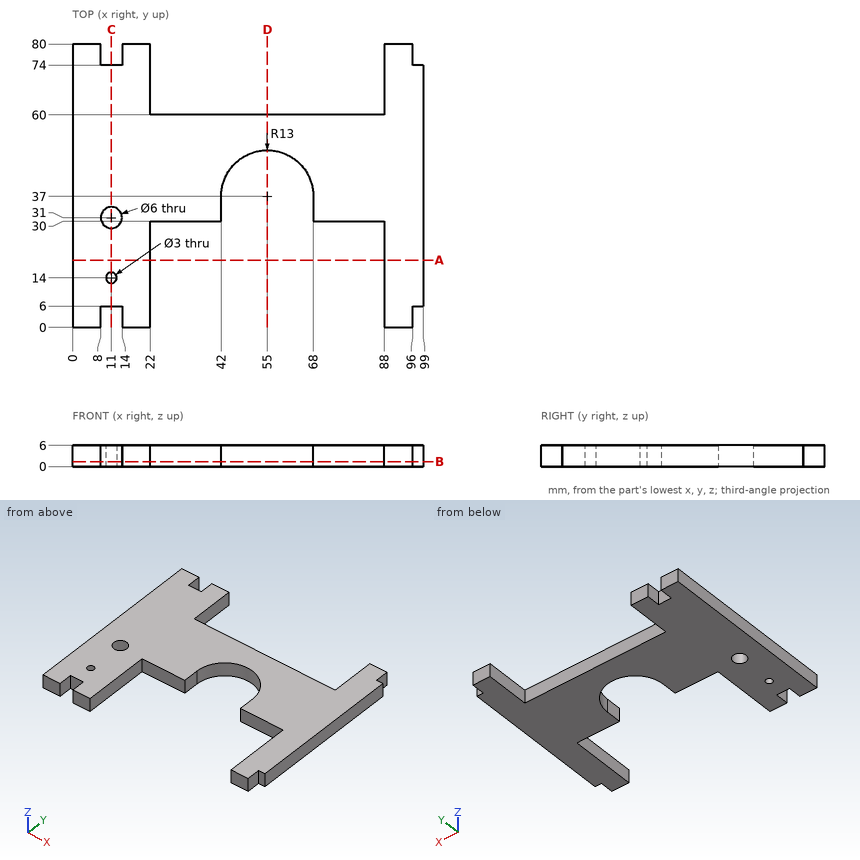
Verification items for this drawing (mm, ordinates from the low corner). Coordinates: 2 decimals unless noted, no trailing zeros. Loops run counter-clockwise (first coordinate to the right, second up) from the corner with the lowest first, then second, coordinate; pieces in that order, holes last. Notation, with made-up numbers: (44.25, -21.75) - (88.25, -21.75) arc R19 ccw to (88.25, -1.75) - close; hole circle Ø9 at (59.25, 23.25). An arc over 180 degrees is marked (long way). Answer as a JSON object with one key per item and string values.
(1) Cross-section at C-C, the plane x = 11. Record the boundary of the cut face in (y, z), then the cut area to 3 significant figures.
Response:
{"outline": "(6, 0) - (12.5, 0) - (12.5, 6) - (6, 6) - close; (15.5, 0) - (28, 0) - (28, 6) - (15.5, 6) - close; (34, 0) - (74, 0) - (74, 6) - (34, 6) - close", "area": "354 mm²"}
(2) Cross-section at B-B, the plane z = 1.4. Count the separate pieces of the cut face and the enclosed holes in it, then the cut area to 3 significant figures.
Response:
{"separate pieces": "1", "enclosed holes": "2", "area": "4,030 mm²"}
(3) Cross-section at A-A, the plane y = 19. Record the boundary of the cut face in (x, z), then the cut area to 3 significant figures.
Response:
{"outline": "(0, 0) - (22, 0) - (22, 6) - (0, 6) - close; (88, 0) - (99, 0) - (99, 6) - (88, 6) - close", "area": "198 mm²"}
(4) Scan lines: line 1 along Y through (x, z) = (11, 4.25); line 2 along X through (y, z) = (77, 5.75); line 3 along X through (y, z) = (63, 3.9). Record each from-to range of solid material in increasing order.
Response:
{"line 1": "y = 6 to 12.5, 15.5 to 28, 34 to 74", "line 2": "x = 0 to 8, 14 to 22, 88 to 96", "line 3": "x = 0 to 22, 88 to 99"}
(5) Cross-section at D-D, the plane x = 55. Record the boundary of the cut face in (y, z), then the cut area to 3 significant figures.
Response:
{"outline": "(50, 0) - (60, 0) - (60, 6) - (50, 6) - close", "area": "60.0 mm²"}
(6) Go/stop test with flat-tipped pins: pin 1 Ø1.8 at (y, z) = (77, 4) entering from +X; pin 2 Ø12 at (x, y) = (45.5, 41.5) entering from -Z; pin 3 Ø2.5 at (x, y) = (11, 14) entering from -Z; pin 4 Ø2 at (x, z) = (37.5, 4) entering from -Y. Record where each tip stops, or that it passes through.
Response:
{"pin 1": "stops at x = 96", "pin 2": "stops at z = 0", "pin 3": "passes through", "pin 4": "stops at y = 30"}
